```python
from build123d import *

# Parameters (mm, degrees)
TABAN_FLAN_1_DEPTH = 15


# Sheet-metal steps are written as plain solids
with BuildPart() as part:
    # Çizim1 → Taban-Flanş1 (new body)
    with BuildSketch(Plane.XY):
        with BuildLine():
            Line((-234.910345825, 161.344850299), (-234.910345825, -238.655149701))
            Line((-234.910345825, -238.655149701), (165.089654175, -238.655149701))
            Line((165.089654175, -238.655149701), (165.089654175, 161.344850299))
            Line((165.089654175, 161.344850299), (96.089654175, 161.344850299))
            Line((96.089654175, 161.344850299), (96.089654175, -3.655149701))
            ThreePointArc((96.089654175, -3.655149701), (85.545498298, -29.110993823), (60.089654175, -39.655149701))
            Line((60.089654175, -39.655149701), (-129.910345825, -39.655149701))
            ThreePointArc((-129.910345825, -39.655149701), (-155.366189948, -29.110993823), (-165.910345825, -3.655149701))
            Line((-165.910345825, -3.655149701), (-165.910345825, 161.344850299))
            Line((-165.910345825, 161.344850299), (-234.910345825, 161.344850299))
        make_face()
    extrude(amount=-TABAN_FLAN_1_DEPTH)


solid = part.part
```
For this review, take the finished solid that the model builds, in its own axes (mm). A direction names the side the tool comes from. Give positions to 0.01 mm unless a question says otherwise; leave off trailing zeros. Write each loop counter-clockwise with the first axis right and the second up, starting at its lowest first coordinate (ties: lowest second). Pieces come first, ordered by that corner, then holes. Notation, with made-up numbers: M -19.5,24.25 L -7.5,24.25 A21 cw -7.5,41.25 Z; hole C 68,-25.75 d10. An arc over 180 degrees is marked long. Answer as a JSON object with one key per item and string values. Group by question number.
Item 1: Consider section C-C on x = 2.5. Write out the cut boundary in (y, z), plus the area to 4 significant figures.
Item 2: For probe 1 along X at (y, z) = (21.5, -8.5); probe 2 along Y at (x, z) = (34, -7.75); probe 3 along X at (y, z) = (-36, -11.5), list the stretches that pass through material, from the lowest coordinate up. Write a range as [from, to].
Item 3: Tool access review of faces 4 (the cylindrical face through (-155.085, -29.389, -7.395)), 5 (the flat face through (165.09, -41, -7)): name each direction out of +Z, -Z, +X, -X, +Y, -Y from which nothing blocks a thin tool from reaching the whole face with its end or side.
Item 4: Consider section A-A on y = 44.5. Write out the cut boundary in (x, z).
Item 5: Draft analysis for pull direction X (two halves, no side actions). For faces 1 (the flat face through (-38, -80, 0)), 2 (the flat face through (-234.91, -36, -7)), 3 (the cylindrical face through (85.824, -28.83, -7.395)), state which applies: +X half, -X half, draft (parallel to the pull), parting line (faces both ways), or undercut.
Item 6: Consider section B-B on z = -10.25. Write out the cut boundary in (x, y).
Item 7: For pin 1 Ø1 at (x, z) = (-80.5, -10.5) entering from +Y, flat-tipped, find the tip position at first contact; note if it passes through.
Check result:
{
 "1": {"outline": "M -238.66,-15 L -39.66,-15 L -39.66,0 L -238.66,0 Z", "area": "2,985 mm^2"},
 "2": {"probe 1": "x = [-234.91, -165.91], [96.09, 165.09]", "probe 2": "y = [-238.66, -39.66]", "probe 3": "x = [-234.91, -145.72], [75.9, 165.09]"},
 "3": {"face 4": "+Z, -Z, +Y", "face 5": "+Z, -Z, +X, +Y, -Y"},
 "4": {"outline": "M -234.91,-15 L -165.91,-15 L -165.91,0 L -234.91,0 Z; M 96.09,-15 L 165.09,-15 L 165.09,0 L 96.09,0 Z"},
 "5": {"face 1": "draft", "face 2": "-X half", "face 3": "undercut"},
 "6": {"outline": "M -234.91,-238.66 L 165.09,-238.66 L 165.09,161.34 L 96.09,161.34 L 96.09,-3.66 A36 cw 60.09,-39.66 L -129.91,-39.66 A36 cw -165.91,-3.66 L -165.91,161.34 L -234.91,161.34 Z"},
 "7": {"pin 1": "stops at y = -39.66"}
}
